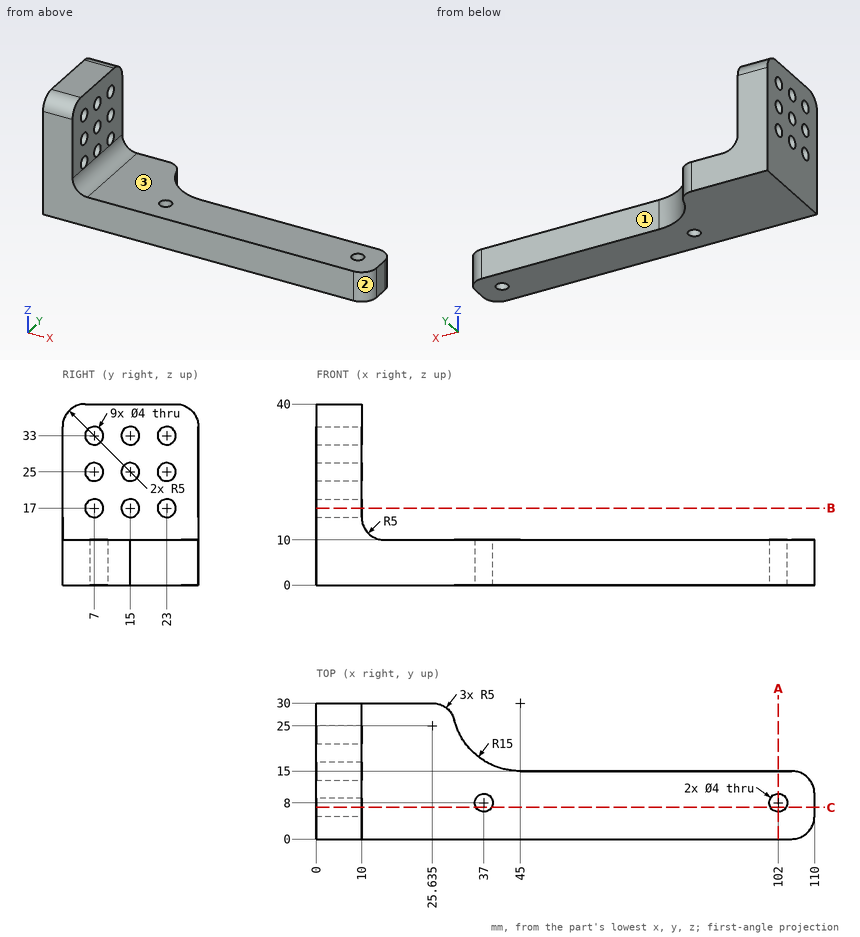
Answer from the drawing. Dimensions are ordinates in mm from the lowest x, y and z of the part. A direction names the side the tool comes from. Round coordinates to 2 decimals unless told otherwise and drop trailing zeros. Loops run counter-clockwise (first coordinate to the right, second up) from the corner with the lowest first, then second, coordinate; pieces in that order, holes last. Notation, with made-up numbers: (68.25, 32.5) - (113.25, 32.5) arc R16 cw to (113.25, 38.5) - close; hole circle Ø11 at (23.25, 60). An arc over 180 degrees is marked (long way). One line per item, written item: value.
Q1. Find section A-A on x = 102. Give the vertices of the cut face in (y, z).
Check values:
outline: (0, 0) - (6, 0) - (6, 10) - (0, 10) - close; (10, 0) - (15, 0) - (15, 10) - (10, 10) - close
Q2. Find section C-C on y = 7. State how many separate pieces and enclosed holes the cut face has, and give its area (3 significant figures).
Check values:
separate pieces: 6
enclosed holes: 0
area: 1,220 mm2
Q3. For the marked faces 1, 2 and 3, determine the directions among +Z, -Z, +X, -X, +Y, -Y from which every point of the face is accessible in a straight line to the end or side of a thin tool.
Check values:
face 1: +Z, -Z, +X, +Y
face 2: +Z, -Z, +X, -Y
face 3: +Z, +X, +Y, -Y
Q4. Each of these flat-tipped pins is pushed along its axis until it touches: pin 1 Ø2.5 at (y, z) = (7, 17) entering from +X; pin 2 Ø5 at (x, z) = (70.5, 2.5) entering from +Y; pin 3 Ø5 at (x, y) = (102, 8) entering from +Z; pin 4 Ø12.5 at (y, z) = (16.5, 31.5) entering from +X. Where does it stop, or does it pass through?
Check values:
pin 1: through
pin 2: y = 15
pin 3: z = 10
pin 4: x = 10
Q5. Straight lines are drawn through the part: probe 1 along Z at (x, y) = (3.5, 7); probe 2 along X at (y, z) = (17.5, 28.5). For each, find the intervals that lie inside material, in ascending order.
Check values:
probe 1: 0 to 15, 19 to 23, 27 to 31, 35 to 40
probe 2: 0 to 10
Q6. Find section B-B on z = 17. Give the vertices of the cut face in (x, y), and give its area (3 significant figures).
Check values:
outline: (0, 0) - (10, 0) - (10, 5) - (0, 5) - close; (0, 9) - (10, 9) - (10, 13) - (0, 13) - close; (0, 17) - (10, 17) - (10, 21) - (0, 21) - close; (0, 25) - (10, 25) - (10, 30) - (0, 30) - close
area: 180 mm2
